Design review of the part shown in the three views and the two pictorial views. Dimensions are in mm from the part's minimum x, y and z. A direction names the side the tool comes from. Round coordinates to 2 decimals unless told otherwise and drop trailing zeros. Order: outer loops, then holes, each group sorted by start corner. A loop starts at its lowest first (then second) coordinate and runs counter-clockwise, first axis right, second up.
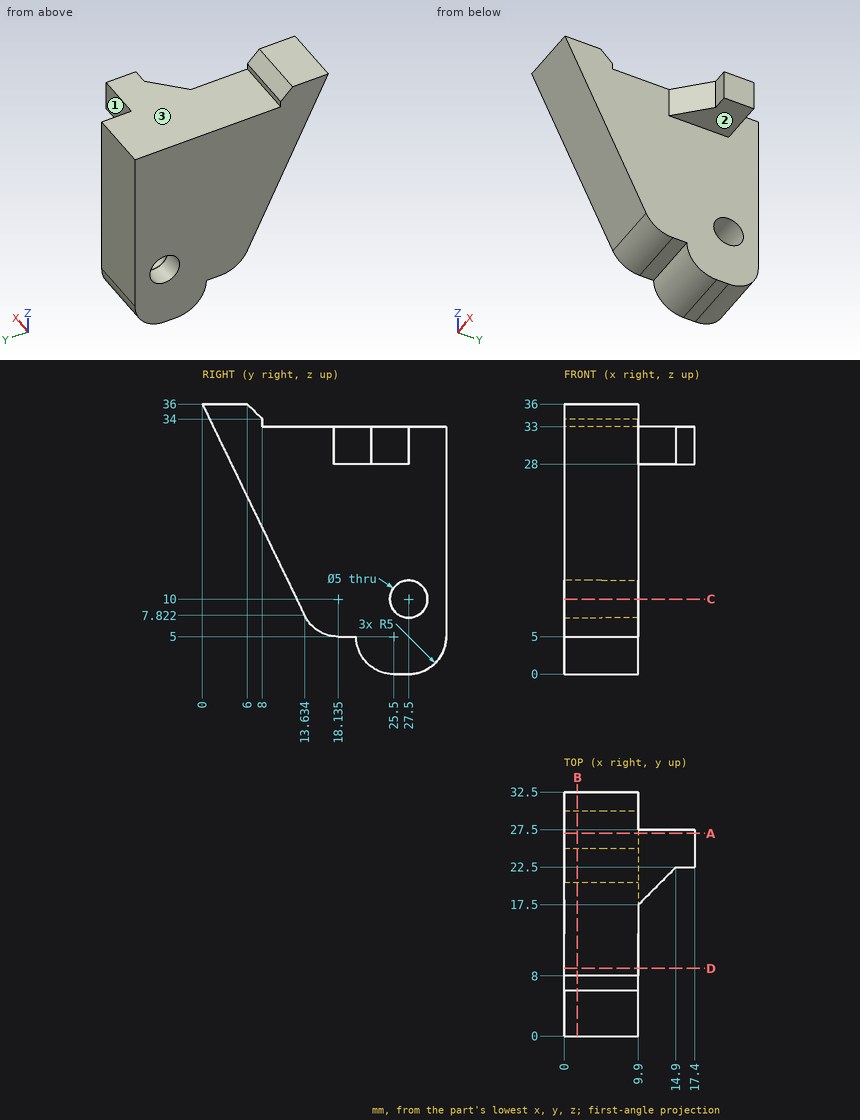
(1) Consider section C-C (z = 10). Write out the cut boundary in (x, y).
Data:
outline: (0, 12.58) - (9.9, 12.58) - (9.9, 25) - (0, 25) - close; (0, 30) - (9.9, 30) - (9.9, 32.5) - (0, 32.5) - close
(2) Consider section B-B (x = 1.75). Write out the cut boundary in (y, z) (1 decimal).
Data:
outline: (0, 36) - (13.6, 7.8) arc R5 ccw to (18.1, 5) - (20.5, 5) arc R5 ccw to (25.5, 0) - (27.5, 0) arc R5 ccw to (32.5, 5) - (32.5, 33) - (8, 33) - (8, 34) - (6, 36) - close; hole circle Ø5 at (27.5, 10)
(3) Consider section D-D (y = 9). Write out the cut boundary in (x, z), and give its area (3 significant figures).
Data:
outline: (0, 17.4) - (9.9, 17.4) - (9.9, 33) - (0, 33) - close
area: 154 mm2
(4) For the marked faces 1, 2 and 3, list the 3-axis set-ups (+Z, -Z, +X, -X, +Y, -Y) from which the entire face can be reached by the end or side of a thin tool; tool diameter is ignored.
Data:
face 1: +Z, -Z, +X, +Y
face 2: -Z, +X, +Y, -Y
face 3: +Z, +X, -X, +Y
(5) Consider section A-A (y = 27). Write out the cut boundary in (x, z).
Data:
outline: (0, 0) - (9.9, 0) - (9.9, 7.55) - (0, 7.55) - close; (0, 12.45) - (9.9, 12.45) - (9.9, 28) - (17.4, 28) - (17.4, 33) - (0, 33) - close
(6) Insertion check: pin 1 (6 mm diameter, centred on x = 5.5, y = 19, fed in from -Z); pin 2 (6 mm diameter, centred on y = 27.5, z = 10, fed in from -X); pin 3 (4 mm diameter, centred on y = 15, z = 25.5, fed in from +X); pin 4 (0.7 mm diameter, centred on x = 3.5, y = 19.5, fed in from -Z). Each pin has a flat end and moves straight along its axis. Give the tip position at first contact, or say it passes through.
Data:
pin 1: stops at z = 1.43
pin 2: stops at x = 0
pin 3: stops at x = 9.9
pin 4: stops at z = 5
(7) To check wall thickness, follow probe 1 along Z at (x, y) = (8.85, 27.5); probe 2 along X at (y, z) = (5, 30); probe 3 along Z at (x, y) = (10.25, 21). State the ranges of each line that lie inside material, in increasing order.
Data:
probe 1: z = 0 to 7.5, 12.5 to 33
probe 2: x = 0 to 9.9
probe 3: z = 28 to 33
